Design review of the part built by this model. Coordinates are the model's own, in mm. A direction names the side the tool comes from. Coordinates: 2 decimals unless noted, no trailing zeros. Loops run counter-clockwise (first coordinate to the right, second up) from the corner with the lowest first, then second, coordinate; pieces in that order, holes last. Notation, with made-up numbers: M -30.75,-2 L 6.25,-2 A5 ccw 6.25,2 Z; hole C 39.5,-30 d5. An arc over 180 degrees is marked long. Put each result on its own line as item: value. Start each with the question number.
(1) Take a section at A-A, the plane x = -53.5. Give the boundary of the cut face in (y, z), then the cut area to 3 significant figures.
(2) For probe 1 along X at (y, z) = (2.3, 15.25) (3 decimals); probe 2 along Z at (x, y) = (-13.5, 2.75); probe 3 along X at (y, z) = (1.45, 59), list the stretches that pass through material, from the lowest coordinate up. Write a range as [from, to].
(3) Clearance check with flat-ended pins moving along their axes: pin 1 (1.9 mm diameter, centred on x = 76.08, z = -58.3, fed in from -Y); pin 2 (1.6 mm diameter, centred on x = 6.5, y = 1, fed in from -Z); pin 3 (1 mm diameter, centred on x = 68, y = 2.5, fed in from -Z). State where each tip first meets the part, or that it passes through.
(4) For faces 4 (the flat face through (47.905, 1.479, -53.251)), 5 (the flat face through (-60.049, 1.479, -37.333)), 6 (the flat face through (59.4, 1.48, -36.79)), list the 3-axis set-ups (+Z, -Z, +X, -X, +Y, -Y) from which the entire face can be reached by the end or side of a thin tool; tool diameter is ignored.
(5) Take a section at B-B, the plane x = -3. Count the separate pieces of the cut face and the enclosed holes in it, then the cut area to 3 significant figures.
(6) The part is to be moulded in two halves that separate along Z. For faces 1 (the flat face through (0, 3, 5)), 2 (the cylindrical face through (-0.38, 1.479, 24.934)), 3 (the flat face through (-59.4, 1.48, 36.79)), say which applies: +Z half, -Z half, draft (parallel to the pull), parting line (faces both ways), or undercut.
```python
from build123d import *

# Parameters (mm, degrees)
SKETCH2_R           = 1.05
SKETCH2_R_2         = 2.75
BOSS_EXTRUDE2_DEPTH = 3
SKETCH4_R           = 1.375
CUT_EXTRUDE1_DEPTH  = 3
CUT_EXTRUDE2_DEPTH  = 3
FILLET3_R           = 0.5


with BuildPart() as part:
    # Sketch2 → Boss-Extrude2 (new body)
    with BuildSketch(Plane(origin=(0, 0, 0), x_dir=(1, 0, 0), z_dir=(0, 1, 0))):
        with BuildLine():
            Line((-83.032320409, 56.618316537), (-36.412926139, 17.5))
            ThreePointArc((-36.412926139, 17.5), (-28.252542121, 0), (-36.412926139, -17.5))
            Line((-36.412926139, -17.5), (-83.032320409, -56.618316537))
            ThreePointArc((-83.032320409, -56.618316537), (-84.264888743, -70.706637066), (-70.176568215, -71.9392054))
            Line((-70.176568215, -71.9392054), (-25, -34.031563673))
            ThreePointArc((-25, -34.031563673), (0, -24.932307816), (25, -34.031563673))
            Line((25, -34.031563673), (70.176568215, -71.9392054))
            ThreePointArc((70.176568215, -71.9392054), (84.264888743, -70.706637066), (83.032320409, -56.618316537))
            Line((83.032320409, -56.618316537), (36.412926139, -17.5))
            ThreePointArc((36.412926139, -17.5), (28.252542121, 0), (36.412926139, 17.5))
            Line((36.412926139, 17.5), (83.032320409, 56.618316537))
            ThreePointArc((83.032320409, 56.618316537), (84.264888743, 70.706637066), (70.176568215, 71.9392054))
            Line((70.176568215, 71.9392054), (25, 34.031563673))
            ThreePointArc((25, 34.031563673), (0, 24.932307816), (-25, 34.031563673))
            Line((-25, 34.031563673), (-70.176568215, 71.9392054))
            ThreePointArc((-70.176568215, 71.9392054), (-84.264888743, 70.706637066), (-83.032320409, 56.618316537))
        make_face()
        with Locations(Location((-77.127378768, 70.255929157, 0), (0, 0, 270))):
            Circle(SKETCH2_R, mode=Mode.SUBTRACT)
        with Locations(Location((-70.627276123, 64.801695425, 0), (0, 0, 270))):
            Circle(SKETCH2_R, mode=Mode.SUBTRACT)
        with Locations(Location((-76.081509855, 58.30159278, 0), (0, 0, 270))):
            Circle(SKETCH2_R, mode=Mode.SUBTRACT)
        with Locations(Location((-82.5816125, 63.755826512, 0), (0, 0, 270))):
            Circle(SKETCH2_R, mode=Mode.SUBTRACT)
        with Locations(Location((-76.604444312, 64.278760969, 0), (0, 0, 270))):
            Circle(SKETCH2_R_2, mode=Mode.SUBTRACT)
        with Locations(Location((-77.127378768, -70.255929157, 0), (0, 0, 90))):
            Circle(SKETCH2_R, mode=Mode.SUBTRACT)
        with Locations(Location((-76.081509855, -58.30159278, 0), (0, 0, 90))):
            Circle(SKETCH2_R, mode=Mode.SUBTRACT)
        with Locations(Location((-82.5816125, -63.755826512, 0), (0, 0, 90))):
            Circle(SKETCH2_R, mode=Mode.SUBTRACT)
        with Locations(Location((-76.604444312, -64.278760969, 0), (0, 0, 90))):
            Circle(SKETCH2_R_2, mode=Mode.SUBTRACT)
        with Locations(Location((-70.627276123, -64.801695425, 0), (0, 0, 90))):
            Circle(SKETCH2_R, mode=Mode.SUBTRACT)
        with Locations(Location((70.627276123, -64.801695425, 0), (0, 0, 270))):
            Circle(SKETCH2_R, mode=Mode.SUBTRACT)
        with Locations(Location((76.604444312, -64.278760969, 0), (0, 0, 270))):
            Circle(SKETCH2_R_2, mode=Mode.SUBTRACT)
        with Locations(Location((82.5816125, -63.755826512, 0), (0, 0, 270))):
            Circle(SKETCH2_R, mode=Mode.SUBTRACT)
        with Locations(Location((76.081509855, -58.30159278, 0), (0, 0, 270))):
            Circle(SKETCH2_R, mode=Mode.SUBTRACT)
        with Locations(Location((77.127378768, -70.255929157, 0), (0, 0, 270))):
            Circle(SKETCH2_R, mode=Mode.SUBTRACT)
        with Locations(Location((76.604444312, 64.278760969, 0), (0, 0, 90))):
            Circle(SKETCH2_R_2, mode=Mode.SUBTRACT)
        with Locations(Location((82.5816125, 63.755826512, 0), (0, 0, 90))):
            Circle(SKETCH2_R, mode=Mode.SUBTRACT)
        with Locations(Location((76.081509855, 58.30159278, 0), (0, 0, 90))):
            Circle(SKETCH2_R, mode=Mode.SUBTRACT)
        with Locations(Location((70.627276123, 64.801695425, 0), (0, 0, 90))):
            Circle(SKETCH2_R, mode=Mode.SUBTRACT)
        with Locations(Location((77.127378768, 70.255929157, 0), (0, 0, 90))):
            Circle(SKETCH2_R, mode=Mode.SUBTRACT)
    extrude(amount=BOSS_EXTRUDE2_DEPTH)

    # Sketch4 → Cut-Extrude1 (cut)
    with BuildSketch(Plane(origin=(0, 0, 0), x_dir=(1, 0, 0), z_dir=(0, 1, 0))):
        with Locations(Location((-15.25, 15.25, 0), (0, 0, 270))):
            Circle(SKETCH4_R)
        with Locations(Location((15.25, -15.25, 0), (0, 0, 270))):
            Circle(SKETCH4_R)
        with Locations(Location((-15.25, -15.25, 0), (0, 0, 270))):
            Circle(SKETCH4_R)
        with Locations(Location((15.25, 15.25, 0), (0, 0, 270))):
            Circle(SKETCH4_R)
    extrude(amount=CUT_EXTRUDE1_DEPTH, mode=Mode.SUBTRACT)

    # Sketch5 → Cut-Extrude2 (cut)
    with BuildSketch(Plane(origin=(0, 3, 0), x_dir=(1, 0, 0), z_dir=(0, 1, 0))):
        with BuildLine():
            Line((-15.25, 20.25), (15.25, 20.25))
            ThreePointArc((15.25, 20.25), (0, 13.189764295), (-15.25, 20.25))
        make_face()
        with BuildLine():
            Line((-15.25, -20.25), (15.25, -20.25))
            ThreePointArc((15.25, -20.25), (0, -13.189764295), (-15.25, -20.25))
        make_face()
    extrude(amount=-CUT_EXTRUDE2_DEPTH, mode=Mode.SUBTRACT)

    # Fillet3
    fillet3_edges = [part.edges().sort_by_distance(p)[0] for p in [
        (0, 0, -13.189764295),
        (0, 0, -20.25),
        (0, 3, -13.189764295),
        (0, 3, -20.25),
        (0, 0, 13.189764295),
        (0, 0, 20.25),
        (0, 3, 13.189764295),
        (0, 3, 20.25),
    ]]
    fillet(fillet3_edges, radius=FILLET3_R)


solid = part.part
```
Computed values:
1. outline: M 0,-57.95 L 3,-57.95 L 3,-31.84 L 0,-31.84 Z; M 0,31.84 L 3,31.84 L 3,57.95 L 0,57.95 Z
1. area: 157 mm^2
2. probe 1: x = [-34.088, -16.625], [-13.875, -8.841], [8.841, 13.875], [16.625, 34.088]
2. probe 2: z = [-27.35, -20.32], [-18.34, 18.34], [20.32, 27.35]
2. probe 3: x = [-85.1, -76.87], [-75.3, -54.76], [54.76, 75.3], [76.87, 85.1]
3. pin 1: passes through
3. pin 2: stops at z = -25.62
3. pin 3: stops at z = -70.53
4. face 4: -Z, +Y, -Y
4. face 5: -X, +Y, -Y
4. face 6: +X, +Y, -Y
5. separate pieces: 3
5. enclosed holes: 0
5. area: 109 mm^2
6. face 1: draft
6. face 2: +Z half
6. face 3: undercut
